from build123d import *

# Parameters (mm, degrees)
SKETCH1_R            = 2.550000000000004
SKETCH1_R_2          = 2.5499999999999914
SKETCH1_R_3          = 2.5500000000000007
SKETCH1_R_4          = 2.550000000000003
BOSS_EXTRUDE1_DEPTH  = 5
BOSS_EXTRUDE2_DEPTH  = 9
BOSS_EXTRUDE3_DEPTH  = 5
BOSS_EXTRUDE4_DEPTH  = 5
SKETCH8_R            = 1.5000000000000009
SKETCH8_R_2          = 1.5000000000000042
SKETCH8_R_3          = 12.000000000000002
CUT_EXTRUDE3_DEPTH   = 115.84184777336179
BOSS_EXTRUDE5_START  = -5
BOSS_EXTRUDE5_DEPTH  = 5
FILLET1_R            = 8
BOSS_EXTRUDE7_START  = 5
BOSS_EXTRUDE7_DEPTH  = 5
CUT_EXTRUDE4_START   = -10
SKETCH12_R           = 1.5500000000000012
SKETCH12_R_2         = 1.5500000000000003
CUT_EXTRUDE4_DEPTH   = 10
SKETCH13_W           = 14.999999999999995
SKETCH13_H           = 15.000000000000043
SKETCH13_R           = 5.0000000000000036
BOSS_EXTRUDE8_DEPTH  = 5
FILLET2_R            = 8
CUT_EXTRUDE5_DEPTH   = 115.92454046025158
SKETCH15_W           = 7.5
SKETCH15_H           = 5.399999999999997
CUT_EXTRUDE6_DEPTH   = 60
SKETCH17_W           = 8
SKETCH17_H           = 7.999999999999998
SKETCH17_R           = 2.999999999999999
BOSS_EXTRUDE10_DEPTH = 3
FILLET4_R            = 3
CHAMFER1_SIZE        = 1
SKETCH18_W           = 8
SKETCH18_H           = 7.999999999999993
SKETCH18_R           = 3
BOSS_EXTRUDE11_DEPTH = 3
FILLET5_R            = 3
CHAMFER2_SIZE        = 1
CUT_EXTRUDE7_DEPTH   = 6


# Some blends are built 0.0001 mm under size
with BuildPart() as part:
    # Sketch1 → Boss-Extrude1 (new body)
    with BuildSketch(Plane.XY):
        with BuildLine():
            Line((0, 0), (33.99999999999999, 0))
            Line((33.99999999999999, 0), (33.99999999999999, 3.0000000000000107))
            ThreePointArc((33.99999999999999, 3.0000000000000107), (32.00000000000001, 7), (33.99999999999999, 10.99999999999999))
            Line((33.99999999999999, 10.99999999999999), (34, 42.7))
            ThreePointArc((34, 42.7), (32, 46.699999999999996), (34, 50.699999999999996))
            Line((34, 50.699999999999996), (34, 53.7))
            Line((34, 53.7), (0, 53.7))
            Line((0, 53.7), (-8.7e-16, 50.7))
            ThreePointArc((-8.7e-16, 50.7), (1.9999999999999938, 46.7), (-8.7e-16, 42.70000000000001))
            Line((-8.7e-16, 42.70000000000001), (-8.7e-16, 10.999999999999995))
            ThreePointArc((-8.7e-16, 10.999999999999995), (1.9999999999999973, 6.9999999999999964), (-8.7e-16, 2.9999999999999982))
            Line((-8.7e-16, 2.9999999999999982), (0, 0))
        make_face()
        with Locations((6.999999999999999, 46.7)):
            Circle(SKETCH1_R, mode=Mode.SUBTRACT)
        with Locations((27, 46.70000000000002)):
            Circle(SKETCH1_R_2, mode=Mode.SUBTRACT)
        with Locations((6.999999999999999, 6.999999999999997)):
            Circle(SKETCH1_R_3, mode=Mode.SUBTRACT)
        with Locations((27.000000000000004, 6.999999999999999)):
            Circle(SKETCH1_R_4, mode=Mode.SUBTRACT)
    extrude(amount=BOSS_EXTRUDE1_DEPTH)

    # Sketch2 → Boss-Extrude2 (add)
    with BuildSketch(Plane.XY.offset(5)):
        Polygon((22.599999999999994, 60), (22.6, 0), (12.600000000000001, 0), (12.599999999999998, 60), align=None)
    extrude(amount=BOSS_EXTRUDE2_DEPTH)

    # Sketch3 → Boss-Extrude3 (add)
    with BuildSketch(Plane.XY.offset(5)):
        Polygon((2.5999999999999983, 5.799999999999998), (2.5999999999999983, -10), (-25.200000000000003, -10.000000000000004), (-25.200000000000006, 5.799999999999998), align=None)
    extrude(amount=BOSS_EXTRUDE3_DEPTH)

    # Sketch6 → Boss-Extrude4 (add, through all)
    with BuildSketch(Plane.XY.offset(5)):
        Polygon((50.6, 102.70000000000002), (7.6, 102.70000000000002), (7.600000000000005, 59.70000000000002), (50.60000000000001, 59.70000000000002), align=None)
        Polygon((50.60000000000001, 59.70000000000002), (7.600000000000005, 59.70000000000002), (0, 53.7), (34, 53.7), align=None)
    extrude(amount=-BOSS_EXTRUDE4_DEPTH)

    # Sketch8 → Cut-Extrude3 (cut, through all)
    with BuildSketch(Plane.XY.offset(5)):
        with Locations((13.299999999999999, 97.00000000000001)):
            Circle(SKETCH8_R)
        with Locations((44.3, 97.00000000000001)):
            Circle(SKETCH8_R_2)
        with Locations((13.300000000000002, 66.00000000000001)):
            Circle(SKETCH8_R)
        with Locations((44.3, 66.00000000000001)):
            Circle(SKETCH8_R_2)
        with Locations((28.8, 81.50000000000001)):
            Circle(SKETCH8_R_3)
    extrude(amount=-CUT_EXTRUDE3_DEPTH, mode=Mode.SUBTRACT)

    # Sketch9 → Boss-Extrude5 (add)
    with BuildSketch(Plane.XY.offset(5).offset(BOSS_EXTRUDE5_START)):
        with BuildLine():
            Line((33.99999999999999, 10.999999999999986), (50.6, 59.70000000000002))
            Line((50.6, 59.70000000000002), (34, 53.7))
            Line((34, 53.7), (34, 50.699999999999996))
            ThreePointArc((34, 50.699999999999996), (39.236067977499786, 51.172135954999575), (42, 46.699999999999996))
            ThreePointArc((42, 46.699999999999996), (39.236067977499786, 42.227864045000416), (34, 42.7))
            Line((34, 42.7), (33.99999999999999, 10.99999999999999))
        make_face()
    extrude(amount=BOSS_EXTRUDE5_DEPTH)

    # Fillet1
    fillet1_edges = [part.edges().sort_by_distance(p)[0] for p in [
        (50.6, 102.70000000000002, 2.5),
        (7.6, 102.70000000000002, 2.5),
    ]]
    fillet(fillet1_edges, radius=FILLET1_R)

    # Sketch11 → Boss-Extrude7 (add)
    with BuildSketch(Plane(origin=(0, 0, 5), x_dir=(-1, 0, 0), z_dir=(0, 0, -1)).offset(BOSS_EXTRUDE7_START)):
        with BuildLine():
            Line((-2.5999999999999983, -10), (-8.37350269189618, 0))
            Line((-8.37350269189618, 0), (0, 0))
            Line((0, 0), (3.47e-15, 2.9999999999999982))
            ThreePointArc((3.47e-15, 2.9999999999999982), (7.999999999999998, 6.9999999999999964), (8.7e-16, 10.999999999999995))
            Line((8.7e-16, 10.999999999999995), (3.52e-15, 13.705401938363094))
            Line((3.52e-15, 13.705401938363094), (25.200000000000006, 5.799999999999998))
            Line((25.200000000000006, 5.799999999999998), (25.200000000000003, -10.000000000000004))
            Line((25.200000000000003, -10.000000000000004), (-2.5999999999999983, -10))
        make_face()
    extrude(amount=-BOSS_EXTRUDE7_DEPTH)

    # Sketch12 → Cut-Extrude4 (cut)
    with BuildSketch(Plane.XY.offset(10).offset(CUT_EXTRUDE4_START)):
        with Locations((-22.400000000000006, -7.2)):
            Circle(SKETCH12_R)
        with Locations((-0.20000000000000182, 2.999999999999998)):
            Circle(SKETCH12_R_2)
    extrude(amount=CUT_EXTRUDE4_DEPTH, mode=Mode.SUBTRACT)

    # Sketch13 → Boss-Extrude8 (add)
    with BuildSketch(Plane.XY.offset(5)):
        with Locations((0.09999999999999964, 81.50000000000003)):
            Rectangle(SKETCH13_W, SKETCH13_H)
        with Locations((0.09999999999999969, 81.50000000000001)):
            Circle(SKETCH13_R, mode=Mode.SUBTRACT)
    extrude(amount=-BOSS_EXTRUDE8_DEPTH)

    # Fillet2
    # the kernel refuses this fillet: 8 mm, written as the material it takes off along each edge
    with BuildSketch(Plane(origin=(-7.399999999999999, 74, 25), x_dir=(1, 0, 0), z_dir=(0, 0, -1))) as fillet2_piece_1:
        with BuildLine():
            CenterArc((FILLET2_R, -FILLET2_R), FILLET2_R, 90, 90)
            Line((-8.9e-16, -FILLET2_R), (0, 0))
            Line((0, 0), (FILLET2_R, 0))
        make_face()
    extrude(amount=45, mode=Mode.SUBTRACT)
    with BuildSketch(Plane(origin=(-7.399999999999999, 89.00000000000004, 25), x_dir=(1, 0, 0), z_dir=(0, 0, -1))) as fillet2_piece_2:
        with BuildLine():
            CenterArc((FILLET2_R, FILLET2_R), FILLET2_R, 180, 90)
            Line((-8.9e-16, FILLET2_R), (0, 0))
            Line((0, 0), (FILLET2_R, 0))
        make_face()
    extrude(amount=45, mode=Mode.SUBTRACT)

    # Sketch14 → Cut-Extrude5 (cut, through all)
    with BuildSketch(Plane.XY.offset(10)):
        Polygon((-18.300000000000004, 1.8999999999999955), (-4.300000000000003, 1.8999999999999972), (-4.300000000000003, -6.1), (-18.300000000000004, -6.100000000000001), align=None)
    extrude(amount=-CUT_EXTRUDE5_DEPTH, mode=Mode.SUBTRACT)

    # Sketch15 → Cut-Extrude6 (cut)
    with BuildSketch(Plane.XZ):
        with Locations((17.65, 9.5)):
            Rectangle(SKETCH15_W, SKETCH15_H)
    extrude(amount=-CUT_EXTRUDE6_DEPTH, mode=Mode.SUBTRACT)

    # Sketch17 → Boss-Extrude10 (add)
    with BuildSketch(Plane(origin=(0, 20, 0), x_dir=(-1, 0, 0), z_dir=(0, -1, 0))):
        with Locations((-17.6, -18)):
            Rectangle(SKETCH17_W, SKETCH17_H)
        with Locations(Location((-17.6, -18, 0), (0, 0, 90))):
            Circle(SKETCH17_R, mode=Mode.SUBTRACT)
    extrude(amount=BOSS_EXTRUDE10_DEPTH)

    # Fillet4
    fillet4_edges = [part.edges().sort_by_distance(p)[0] for p in [
        (21.6, 18.5, 22),
        (13.600000000000001, 18.5, 22),
    ]]
    fillet(fillet4_edges, radius=FILLET4_R)

    # Chamfer1
    chamfer1_edges = [part.edges().sort_by_distance(p)[0] for p in [
        (17.6, 17, 14.000000000000002),
        (17.6, 20, 14.000000000000002),
    ]]
    chamfer(chamfer1_edges, length=CHAMFER1_SIZE - 0.0001)  # a hair under: the kernel refuses the full size

    # Sketch18 → Boss-Extrude11 (add)
    with BuildSketch(Plane.ZY.offset(-7.600000000000001)):
        with Locations((9.000000000000002, 35.999999999999986)):
            Rectangle(SKETCH18_W, SKETCH18_H)
        with Locations(Location((9.000000000000002, 35.99999999999999, 0), (0, 0, 270))):
            Circle(SKETCH18_R, mode=Mode.SUBTRACT)
    extrude(amount=BOSS_EXTRUDE11_DEPTH)

    # Fillet5
    fillet5_edges = [part.edges().sort_by_distance(p)[0] for p in [
        (6.1, 31.999999999999993, 13.000000000000002),
        (6.099999999999999, 39.999999999999986, 13.000000000000002),
    ]]
    fillet(fillet5_edges, radius=FILLET5_R)

    # Chamfer2
    chamfer2_edges = [part.edges().sort_by_distance(p)[0] for p in [
        (4.6, 35.999999999999986, 5.000000000000001),
        (7.6, 35.999999999999986, 5.000000000000001),
        (6.099999999999999, 39.999999999999986, 5.000000000000001),
        (6.1, 31.999999999999993, 5.000000000000001),
    ]]
    chamfer(chamfer2_edges, length=CHAMFER2_SIZE)

    # Sketch19 → Cut-Extrude7 (cut)
    with BuildSketch(Plane(origin=(0, 0, 0), x_dir=(-1, 0, 0), z_dir=(0, 0, -1))):
        Polygon((25.200000000000003, -10.000000000000004), (18.300000000000004, -10.000000000000004), (18.300000000000008, -3.1000000000000036), (25.200000000000006, -3.1000000000000028), align=None)
    extrude(amount=-CUT_EXTRUDE7_DEPTH, mode=Mode.SUBTRACT)


solid = part.part
Here's how the part is built. I have some questions about the finished solid (model axes, mm). A direction names the side the tool comes from. Round coordinates to 2 decimals unless told otherwise and drop trailing zeros. Loops run counter-clockwise (first coordinate to the right, second up) from the corner with the lowest first, then second, coordinate; pieces in that order, holes last. Notation, with made-up numbers: M 43,65.5 L 56,65.5 A5 cw 56,73.5 Z; hole C 82.5,24.5 d1. An arc over 180 degrees is marked long. Write each question's results on one line, items separated by ' | '. Start each with the question number.
(1) I want a section at D-D (y = 7). Please give me the cut outline in (x, z).
(2) Will these pins go through, and if not, where does the flat tip stop? P1, Ø5, axis at x = -12, z = 4.5, coming from the +Y side; P2, Ø6, axis at x = 11, z = 18, coming from the -Y side; P3, Ø4.5, axis at x = 7, y = 7, coming from the +Z side; P4, Ø6, axis at y = 31.5, z = 8.5, coming from the +X side.
(3) On a 3-axis mill with a long thin cutter (end or side, diameter ignored), from which of +Z, -Z, +X, -X, +Y, -Y can I reach the whole of each face in a straight line? I mean faces 4 (the flat face through (21.4, 30, 9)), 5 (the flat face through (-18.3, -8, 3)), 6 (the flat face through (19, 0, 4)), 7 (the flat face through (-3, 4, 5)), 8 (the cylindrical face through (6.08, 39.14, 12.1)). Say none if no direction works.
(4) If I drill on probe 1 along Z at (x, y) = (17, 19); probe 2 along Y at (x, z) = (13.3, 3.65); probe 3 along Y at (x, z) = (2.5, 3.75), over which ranges is the centre line in solid material (lowest first)? Write a range as from..to.
(5) I want a section at C-C (x = -3). Please give me the cut outline in (y, z).
(6) Thinking about a two-plate mould opening in X: for faces 1 (the flat face through (-4.3, -2, 5)), 2 (the cylindrical face through (-4.94, 86.77, 2.54)), 3 (the flat face through (-11, -10, 5)), which applies, pulls with the +X half, pulls with the -X half, needs draft (parallel to the pull), parting line crosses it, or undercut?
(7) I want a section at B-B (y = 92). Please give me the cut outline in (x, z), then the cut area to 3 significant figures.
(8) I want a section at A-A (x = -16). Please give me the cut outline in (y, z).
Solved:
1) outline: M -21.37,0 L -8,0 L -8,5 L -21.37,5 Z; M 2,0 L 4.45,0 L 4.45,5 L 2,5 Z; M 9.55,0 L 24.45,0 L 24.45,5 L 22.6,5 L 22.6,14 L 12.6,14 L 12.6,5 L 9.55,5 Z; M 29.55,0 L 32,0 L 32,5 L 29.55,5 Z; hole M 13.9,6.8 L 21.4,6.8 L 21.4,12.2 L 13.9,12.2 Z
2) P1: stops at y = 10.73 | P2: stops at y = 17 | P3: passes through | P4: stops at x = 22.6
3) face 4: +Y, -Y | face 5: -Z, -X, -Y | face 6: +Z, -Z, +X, -Y | face 7: -Z | face 8: +Z, -X, +Y
4) probe 1: z = 0..6.8, 12.2..15.06, 20.94..22 | probe 2: y = 0..64.5, 67.5..95.5, 98.5..102.36 | probe 3: y = -10..55.67, 74..77.11, 85.89..89
5) outline: M -10,0 L 2,0 L 2,5 L 5.8,5 L 5.8,10 L -10,10 Z; M 12,0 L 12.76,0 L 12.76,5 L 12,5 Z; M 74.86,0 L 77.58,0 L 77.58,5 L 74.86,5 Z; M 85.42,0 L 88.14,0 L 88.14,5 L 85.42,5 Z
6) face 1: undercut | face 2: pulls with the -X half | face 3: needs draft
7) outline: M 7.6,0 L 22.99,0 L 22.99,5 L 7.6,5 Z; M 34.61,0 L 50.6,0 L 50.6,5 L 34.61,5 Z | area: 157 mm²
8) outline: M -10,0 L -6.1,0 L -6.1,10 L -10,10 Z; M 1.9,0 L 8.69,0 L 8.69,5 L 5.8,5 L 5.8,10 L 1.9,10 Z
